```python
from build123d import *

# Parameters (mm, degrees)
SKETCH1_W                  = 381
SKETCH1_H                  = 193.675
BOSS_EXTRUDE1_DEPTH        = 1.5
CUT_EXTRUDE1_DEPTH         = 214.72120018
CUT_EXTRUDE1_DEPTH_BACK    = 214.72120018
SKETCH2_W                  = 25.4
SKETCH2_H                  = 19.05
SKETCH2_W_2                = 22.225
SKETCH3_W                  = 19.05
SKETCH3_H                  = 12.7
BOSS_EXTRUDE2_DEPTH        = 3
FILLET1_R                  = 3.175
FILLET1_OF_MIRROR1_R       = 3.175
FILLET2_R                  = 1.5875
LPATTERN1_START            = -1.5
LPATTERN1_DEPTH            = 3
F_1_0MM_DOWEL_HOLE6_D      = 6
F_1_0MM_DOWEL_HOLE5_D      = 6
SKETCH10_R                 = 7.75
CUT_EXTRUDE2_DEPTH         = 231.862954816
F_8_CLEARANCE_HOLE1_D      = 4.4958
F_1_0MM_DOWEL_HOLE1_D      = 4.8
F_1_0_4_8_DIAMETER_HOLE1_D = 4.8


# Read off the part's stored shape, not the designer's step: LPattern1
with BuildPart() as part:
    # Sketch1 → Boss-Extrude1 (new, symmetric)
    with BuildSketch(Plane.XY):
        Rectangle(SKETCH1_W, SKETCH1_H)
    extrude(amount=BOSS_EXTRUDE1_DEPTH, both=True)

    # Sketch2 → Cut-Extrude1 (cut, two sides: drawn at the far end of the back side and taken through both)
    with BuildSketch(Plane.XY.offset(1.5).offset(-CUT_EXTRUDE1_DEPTH_BACK)):
        with Locations((-177.8, 87.3125)):
            Rectangle(SKETCH2_W, SKETCH2_H)
        with Locations((80.9625, 87.3125)):
            Rectangle(SKETCH2_W_2, SKETCH2_H)
    extrude(amount=CUT_EXTRUDE1_DEPTH + CUT_EXTRUDE1_DEPTH_BACK, mode=Mode.SUBTRACT)

    # Sketch3 → Boss-Extrude2 (add)
    with BuildSketch(Plane.XY.offset(1.5)):
        with Locations((-200.025, -9.525)):
            Rectangle(SKETCH3_W, SKETCH3_H)
    boss_extrude2 = extrude(amount=-BOSS_EXTRUDE2_DEPTH)

    # Fillet1
    fillet1_edges = [part.edges().sort_by_distance(p)[0] for p in [
        (-209.55, -3.175, 0),
        (-209.55, -15.875, 0),
    ]]
    fillet(fillet1_edges, radius=FILLET1_R)

    # Mirror1: Boss-Extrude2 across plane
    add(boss_extrude2.mirror(Plane(origin=(0, 0, 0), x_dir=(0, 0, 1), z_dir=(1, 0, 0))))

    # Fillet1 of Mirror1
    fillet1_of_mirror1_edges = [part.edges().sort_by_distance(p)[0] for p in [
        (209.55, -3.175, 0),
        (209.55, -15.875, 0),
    ]]
    fillet(fillet1_of_mirror1_edges, radius=FILLET1_OF_MIRROR1_R)

    # Fillet2
    fillet2_edges = [part.edges().sort_by_distance(p)[0] for p in [
        (-190.5, -15.875, 0),
        (-190.5, -3.175, 0),
        (190.5, -15.875, 0),
        (190.5, -3.175, 0),
    ]]
    fillet(fillet2_edges, radius=FILLET2_R)

    # LPattern1 outline → LPattern1 (add)
    with BuildSketch(Plane.XY.offset(LPATTERN1_START)):
        with BuildLine():
            ThreePointArc((-206.375, 47.625), (-208.62006403, 46.69506403), (-209.55, 44.45))
            Line((-209.55, 44.45), (-209.55, 38.1))
            ThreePointArc((-209.55, 38.1), (-208.62006403, 35.85493597), (-206.375, 34.925))
            Line((-206.375, 34.925), (-192.0875, 34.925))
            ThreePointArc((-192.0875, 34.925), (-190.964967985, 34.460032015), (-190.5, 33.3375))
            Line((-190.5, 33.3375), (-190.5, 49.2125))
            ThreePointArc((-190.5, 49.2125), (-190.964967985, 48.089967985), (-192.0875, 47.625))
            Line((-192.0875, 47.625), (-206.375, 47.625))
        make_face()
        with BuildLine():
            ThreePointArc((-206.375, -53.975), (-208.62006403, -54.90493597), (-209.55, -57.15))
            Line((-209.55, -57.15), (-209.55, -63.5))
            ThreePointArc((-209.55, -63.5), (-208.62006403, -65.74506403), (-206.375, -66.675))
            Line((-206.375, -66.675), (-192.0875, -66.675))
            ThreePointArc((-192.0875, -66.675), (-190.964967985, -67.139967985), (-190.5, -68.2625))
            Line((-190.5, -68.2625), (-190.5, -52.3875))
            ThreePointArc((-190.5, -52.3875), (-190.964967985, -53.510032015), (-192.0875, -53.975))
            Line((-192.0875, -53.975), (-206.375, -53.975))
        make_face()
        with BuildLine():
            Line((209.55, 38.1), (209.55, 44.45))
            ThreePointArc((209.55, 44.45), (208.62006403, 46.69506403), (206.375, 47.625))
            Line((206.375, 47.625), (192.0875, 47.625))
            ThreePointArc((192.0875, 47.625), (190.964967985, 48.089967985), (190.5, 49.2125))
            Line((190.5, 49.2125), (190.5, 33.3375))
            ThreePointArc((190.5, 33.3375), (190.964967985, 34.460032015), (192.0875, 34.925))
            Line((192.0875, 34.925), (206.375, 34.925))
            ThreePointArc((206.375, 34.925), (208.62006403, 35.85493597), (209.55, 38.1))
        make_face()
        with BuildLine():
            Line((209.55, -63.5), (209.55, -57.15))
            ThreePointArc((209.55, -57.15), (208.62006403, -54.90493597), (206.375, -53.975))
            Line((206.375, -53.975), (192.0875, -53.975))
            ThreePointArc((192.0875, -53.975), (190.964967985, -53.510032015), (190.5, -52.3875))
            Line((190.5, -52.3875), (190.5, -68.2625))
            ThreePointArc((190.5, -68.2625), (190.964967985, -67.139967985), (192.0875, -66.675))
            Line((192.0875, -66.675), (206.375, -66.675))
            ThreePointArc((206.375, -66.675), (208.62006403, -65.74506403), (209.55, -63.5))
        make_face()
    extrude(amount=LPATTERN1_DEPTH)

    # Ø1.0mm Dowel Hole6 (through all)
    with Locations(Plane.XY.offset(1.5)):
        with Locations((114.080868605, -1.328387664)):
            Hole(F_1_0MM_DOWEL_HOLE6_D / 2)

    # Ø1.0mm Dowel Hole5 (through all)
    with Locations(Plane.XY.offset(1.5)):
        with Locations((62.931618599, -25.649221104)):
            Hole(F_1_0MM_DOWEL_HOLE5_D / 2)

    # Sketch10 → Cut-Extrude2 (cut, through all)
    with BuildSketch(Plane.XY.offset(1.5)):
        with Locations((86.013868605, 9.09694676)):
            Circle(SKETCH10_R)
    extrude(amount=-CUT_EXTRUDE2_DEPTH, mode=Mode.SUBTRACT)

    # #8 Clearance Hole1 (through all)
    with Locations(Plane(origin=(0, 0, -1.5), x_dir=(-1, 0, 0), z_dir=(0, 0, -1))):
        with Locations((3.488631395, 16.97194676), (-28.261368605, 16.97194676), (-28.261368605, -14.77805324), (3.488631395, -14.77805324), (-56.930868605, -87.847137664), (-114.080868605, -87.847137664), (-171.230868605, -87.847137664), (-165.723368605, 27.246612336), (-181.598368605, 27.246612336), (-181.598368605, -31.490887664), (-165.723368605, -31.490887664), (176.53, 66.736172691), (-97.1296, 88.08565122), (-141.5796, 62.4224304), (165.1, -71.4375)):
            Hole(F_8_CLEARANCE_HOLE1_D / 2)

    # Ø1.0mm Dowel Hole1 (through all)
    with Locations(Plane.XY.offset(1.5)):
        with Locations((-158.944770876, 59.513399002), (-48.646302539, 40.064803103), (-103.795536708, 49.789101052), (-41.555686717, 38.814536224), (13.593547451, 29.090238275), (68.74278162, 19.365940325), (67.618368605, 10.356435791), (67.618368605, -5.643564209), (155.263089531, -18.7625), (155.263089531, 93.2375), (168.480868605, -71.388387664), (168.480868605, -39.388387664)):
            Hole(F_1_0MM_DOWEL_HOLE1_D / 2)

    # Ø1.0 (4.8) Diameter Hole1 (through all)
    with Locations(Plane.XY.offset(1.5)):
        with Locations((196.65, -9.525)):
            Hole(F_1_0_4_8_DIAMETER_HOLE1_D / 2)


solid = part.part
```
Part model, mm, in its own coordinate system. Give positions to 0.01 mm unless a question says otherwise; leave off trailing zeros. Put each result on its own line as item: value. Start each with the question number.
Item 1: Pull direction X, two halves, no side cores. Call faces 1 (the face through (93.173, 6.129, 0.021)), 2 (the face through (-3, 1, 1.5)): pulls with the +X half, pulls with the -X half, needs draft (parallel to the pull), parting line crosses it, or undercut.
Item 2: Cut at A-A (z = 0.05). State how many separate pieces and enclosed holes the cut face has, then the cut area to 3 significant figures.
Item 3: Pin check, flat tips, straight feed: pin 1 Ø2.5 at (x, y) = (114.08, -87.85) entering from +Z; pin 2 Ø0.9 at (x, z) = (202.5, 0.5) entering from +Y (3 decimals); pin 3 Ø0.9 at (x, z) = (-197, 0.5) entering from -Y (3 decimals); pin 4 Ø1.5 at (y, z) = (84, 0.5) entering from -X. Stop position of each tip, or through.
Item 4: Wall check: L1, parallel to Y at x = 155, z = -1.1; L2, parallel to Y at x = 113.5, z = 0.7; L3, parallel to X at y = -87, z = 0.9. Give the ranges that are in metal, low to high. Write a range as [from, to].
Answer list:
1. face 1: undercut
1. face 2: needs draft
2. separate pieces: 1
2. enclosed holes: 31
2. area: 73,600 mm2
3. pin 1: passes through
3. pin 2: stops at y = 47.625
3. pin 3: stops at y = -66.675
3. pin 4: stops at x = -165.1
4. L1: y = [-96.84, -21.15], [-16.38, 90.85], [95.62, 96.84]
4. L2: y = [-96.84, -90.02], [-85.68, -4.27], [1.61, 96.84]
4. L3: x = [-190.5, 54.85], [59.01, 112], [116.16, 169.15], [173.31, 190.5]
